Could you check a few things on this drawing? It's one solid part, dimensions in mm from its lowest x, y, z. A direction names the side the tool comes from. Give positions to 0.01 mm unless a question says otherwise; leave off trailing zeros. Write each loop counter-clockwise with the first axis right and the second up, starting at its lowest first coordinate (ties: lowest second). Pieces come first, ordered by that corner, then holes. Notation, with made-up numbers: M -24,-31 L 0,-31 A32 ccw 0,4 Z; hole C 33,34.25 d6. An arc over 180 degrees is marked long. Answer as CSV lines item,"result". Start each with the question number.
Q1. Suppose I cut it at C-C (z = 52.5). Write out the boundary of the cut face in (x, y), then the cut area to 3 significant figures.
Q2. Suppose I cut it at D-D (x = 36.5). Write out the boundary of the cut face in (y, z).
Q3. For pin 1 (0.8 mm diameter, centred on y = 4.5, z = 57.5, fed in from -X); pin 2 (10 mm diameter, centred on x = 28.5, z = 16.5, fed in from +Y); pin 3 (13.5 mm diameter, centred on x = 18.5, z = 28, fed in from +Y), each with a flat end and sliding along its axis, tell me the tip position at first contact or that it passes through.
Q4. Thinking about a two-plate mould opening in Z: for the marked faces 1, 2, 3 and 4, which applies, +Z half, -Z half, draft (parallel to the pull), parting line (faces both ways), or undercut?
Q5. Suppose I cut it at B-B (y = 9.5). Write out the boundary of the cut face in (x, z).
Q6. If I drill on line 1 along X through (y, z) = (10.5, 14); line 2 along Z through (x, y) = (35, 10); line 3 along Z through (x, y) = (14.5, 4.25), over which ranges is the centre line in solid material (lowest first)?
Q7. Suppose I cut it at A-A (x = 26.5). Write out the boundary of the cut face in (y, z).
Q8. On a 3-axis mill with a long thin cutter (end or side, diameter ignored), from which of +Z, -Z, +X, -X, +Y, -Y can I reach the whole of each face in a straight line? I mean the marked faces 5 and 6. Say none if no direction works.
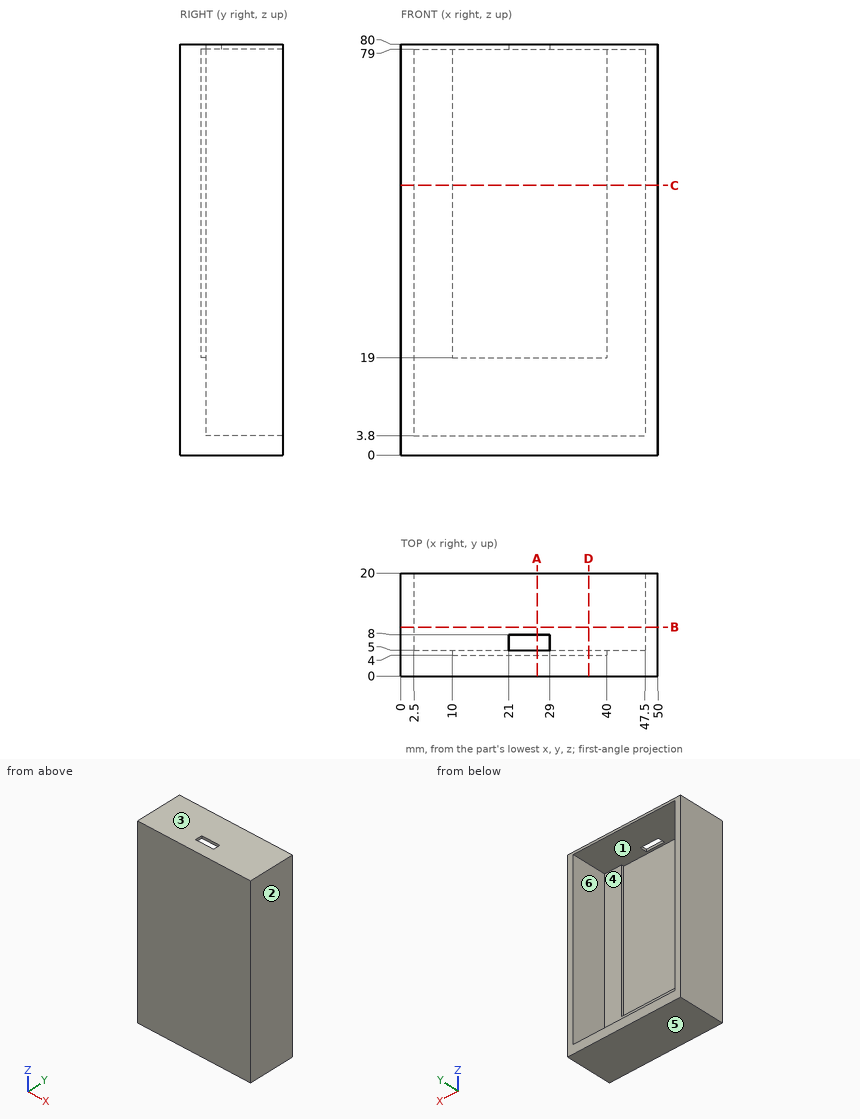
Resolved:
1,outline,"M 0,0 L 50,0 L 50,20 L 47.5,20 L 47.5,5 L 40,5 L 40,4 L 10,4 L 10,5 L 2.5,5 L 2.5,20 L 0,20 Z"
1,area,"295 mm^2"
2,outline,"M 0,0 L 20,0 L 20,3.8 L 5,3.8 L 5,19 L 4,19 L 4,79 L 20,79 L 20,80 L 0,80 Z"
3,pin 1,"x = 0"
3,pin 2,"y = 5"
3,pin 3,"y = 4"
4,face 1,"undercut"
4,face 2,"draft"
4,face 3,"+Z half"
4,face 4,"undercut"
5,outline,"M 0,0 L 50,0 L 50,80 L 0,80 Z; hole M 2.5,3.8 L 47.5,3.8 L 47.5,79 L 2.5,79 Z"
6,line 1,"0 to 2.5, 47.5 to 50"
6,line 2,"0 to 3.8, 79 to 80"
6,line 3,"0 to 19, 79 to 80"
7,outline,"M 0,0 L 20,0 L 20,3.8 L 5,3.8 L 5,19 L 4,19 L 4,79 L 5,79 L 5,80 L 0,80 Z; M 8,79 L 20,79 L 20,80 L 8,80 Z"
8,face 5,"-Z, +X, -X, +Y, -Y"
8,face 6,"+Y"
